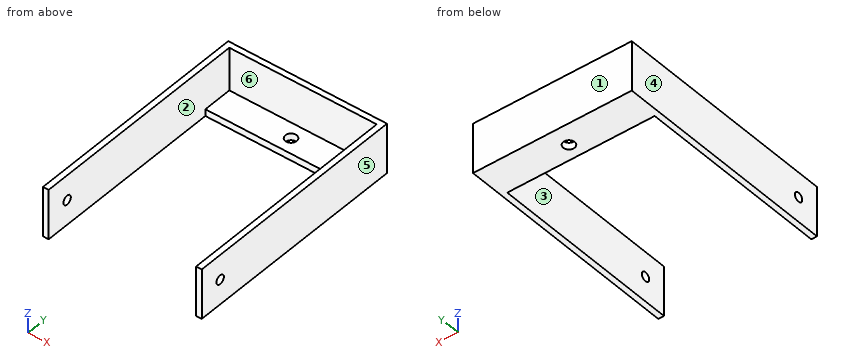
from build123d import *

# Parameters (mm, degrees)
CROQUIS1_W                 = 22
CROQUIS1_H                 = 100.5
CROQUIS1_R                 = 2
SALIENTE_EXTRUIR1_DEPTH    = 35
CORTAR_EXTRUIR2_DEPTH      = 100.494974747
CORTAR_EXTRUIR2_DEPTH_BACK = 100.494974747
CROQUIS3_W                 = 65
CROQUIS3_H                 = 13
CROQUIS3_R                 = 2.5
SALIENTE_EXTRUIR3_DEPTH    = 3


with BuildPart() as part:
    # Croquis1 → Saliente-Extruir1 (new, symmetric)
    with BuildSketch(Plane(origin=(0, 0, 0), x_dir=(0, 0, -1), z_dir=(1, 0, 0))):
        with Locations((0, 40.25)):
            Rectangle(CROQUIS1_W, CROQUIS1_H)
        Circle(CROQUIS1_R, mode=Mode.SUBTRACT)
    extrude(amount=SALIENTE_EXTRUIR1_DEPTH, both=True)

    # Croquis2 → Cortar-Extruir2 (cut, two sides: drawn at the far end of the back side and taken through both)
    with BuildSketch(Plane.XY.offset(11).offset(-CORTAR_EXTRUIR2_DEPTH_BACK)):
        Polygon((32.5, -262.128065288), (32.5, -10), (32.5, 88), (-32.5, 88), (-32.5, -10), (-32.5, -262.128065288), (-32.5, -766.384195863), (32.5, -766.384195863), align=None)
    extrude(amount=CORTAR_EXTRUIR2_DEPTH + CORTAR_EXTRUIR2_DEPTH_BACK, mode=Mode.SUBTRACT)

    # Croquis3 → Saliente-Extruir3 (add)
    with BuildSketch(Plane(origin=(0, 0, -11), x_dir=(-1, 0, 0), z_dir=(0, 0, -1))):
        with Locations((0, 81.5)):
            Rectangle(CROQUIS3_W, CROQUIS3_H)
        with Locations(Location((0, 81.5, 0), (0, 0, 90))):
            Circle(CROQUIS3_R, mode=Mode.SUBTRACT)
    extrude(amount=-SALIENTE_EXTRUIR3_DEPTH)


solid = part.part
Could you check a few things on this model? Use its own coordinates, in mm. Face numbers are marked on the shaded views. A direction names the side the tool comes from. Give positions to 0.01 mm unless a question says otherwise; leave off trailing zeros. Order: outer loops, then holes, each group sorted by start corner. A loop starts at its lowest first (then second) coordinate and runs counter-clockwise, first axis right, second up.
1. Suppose I cut it at B-B (x = 0). Write out the boundary of the cut face in (y, z), plus the area to 3 significant figures.
Answers below:
outline: (75, -11) - (79, -11) - (79, -8) - (75, -8) - close; (84, -11) - (90.5, -11) - (90.5, 11) - (88, 11) - (88, -8) - (84, -8) - close
area: 79.0 mm2
2. Which directions (+Z, -Z, +X, -X, +Y, -Y) give clear straight access to the entire face, cutting with the end or side of a thin tool? Please do the marked faces 5 and 6.
Answers below:
face 5: +Z, -Z, +X, +Y, -Y
face 6: +Z, -Y
3. Suppose I cut it at A-A (y = 69.5). Write out the boundary of the cut face in (x, z).
Answers below:
outline: (-35, -11) - (-32.5, -11) - (-32.5, 11) - (-35, 11) - close; (32.5, -11) - (35, -11) - (35, 11) - (32.5, 11) - close
4. I need wall thicknesses on L1, parallel to X at y = 5.5, z = 1.5; L2, parallel to X at y = 81.5, z = -9.85; L3, parallel to Y at x = -28, z = 5. Which ranges of each line are inside material? Lowest first, please.
Answers below:
L1: x = -35 to -32.5, 32.5 to 35
L2: x = -35 to -2.5, 2.5 to 35
L3: y = 88 to 90.5
5. Suppose I cut it at D-D (y = 0). Write out the boundary of the cut face in (x, z).
Answers below:
outline: (-35, -11) - (-32.5, -11) - (-32.5, -2) - (-35, -2) - close; (-35, 2) - (-32.5, 2) - (-32.5, 11) - (-35, 11) - close; (32.5, -11) - (35, -11) - (35, -2) - (32.5, -2) - close; (32.5, 2) - (35, 2) - (35, 11) - (32.5, 11) - close
6. For pin 1 (10.5 mm diameter, centred on x = -1.5, y = 80.5, fed in from +Z); pin 2 (1.5 mm diameter, centred on x = 19, z = 3.5, fed in from -Y); pin 3 (3.5 mm diameter, centred on x = -6, z = -9.5, fed in from -Y), each with a flat end and sliding along its axis, tell me the tip position at first contact or that it passes through.
Answers below:
pin 1: stops at z = -8
pin 2: stops at y = 88
pin 3: stops at y = 75
7. Suppose I cut it at C-C (z = 0). Write out the boundary of the cut face in (x, y), plus the area to 3 significant figures.
Answers below:
outline: (-35, -10) - (-32.5, -10) - (-32.5, -2) - (-35, -2) - close; (-35, 2) - (-32.5, 2) - (-32.5, 88) - (32.5, 88) - (32.5, 2) - (35, 2) - (35, 90.5) - (-35, 90.5) - close; (32.5, -10) - (35, -10) - (35, -2) - (32.5, -2) - close
area: 645 mm2
8. Thinking about a two-plate mould opening in X: for the marked faces 1, 2, 3 and 4, which applies, +X half, -X half, draft (parallel to the pull), parting line (faces both ways), or undercut?
Answers below:
face 1: draft
face 2: undercut
face 3: undercut
face 4: -X half
